Read the model definition and answer for the solid it produces. Units are mm, in the model's axes. Face numbers are marked on the shaded views. A direction names the side the tool comes from. Round coordinates to 2 decimals unless told otherwise and drop trailing zeros. Write each loop counter-clockwise with the first axis right and the second up, starting at its lowest first coordinate (ties: lowest second). Pieces come first, ordered by that corner, then holes. Notation, with made-up numbers: (22, -18) -> (51, -18) arc R26 cw to (51, -4) -> close; hole circle Ø8 at (64.5, 82). An arc over 180 degrees is marked (long way). Return JSON: item names as keys, results as strings.
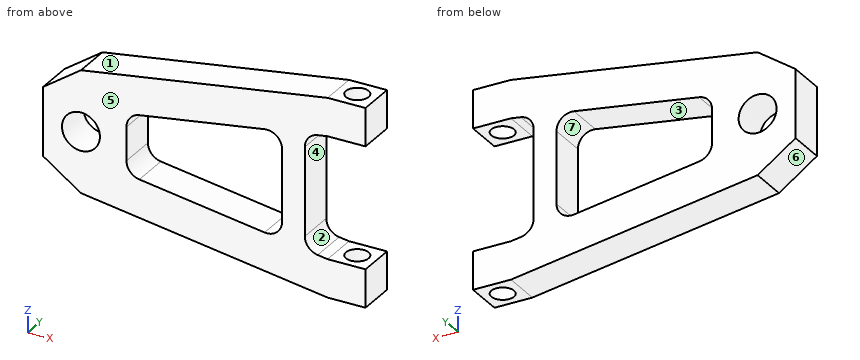
from build123d import *

# Parameters (mm, degrees)
SKETCH1_R           = 2.5
BOSS_EXTRUDE1_DEPTH = 5
SKETCH2_R           = 1.5
CUT_EXTRUDE1_DEPTH  = 46.904792778


with BuildPart() as part:
    # Sketch1 → Boss-Extrude1 (new body)
    with BuildSketch(Plane(origin=(0, 0, 0), x_dir=(1, 0, 0), z_dir=(0, 1, 0))):
        with BuildLine():
            Line((0, 8), (-5, 4.498962309))
            Line((-5, 4.498962309), (-5, -4.498962309))
            Line((-5, -4.498962309), (0, -8))
            Line((0, -8), (32.5, -13))
            Line((32.5, -13), (37.5, -13))
            Line((37.5, -13), (37.5, -8))
            Line((37.5, -8), (32.5, -8))
            Line((32.5, -8), (31.195885631, -7.79936702))
            ThreePointArc((31.195885631, -7.79936702), (29.98206905, -7.124885362), (29.5, -5.822623625))
            Line((29.5, -5.822623625), (29.5, 5.822623625))
            ThreePointArc((29.5, 5.822623625), (29.98206905, 7.124885362), (31.195885631, 7.79936702))
            Line((31.195885631, 7.79936702), (32.5, 8))
            Line((32.5, 8), (37.5, 8))
            Line((37.5, 8), (37.5, 13))
            Line((37.5, 13), (32.5, 13))
            Line((32.5, 13), (0, 8))
        make_face()
        with Locations(Location((0, 0, 0), (0, 0, 270))):
            Circle(SKETCH1_R, mode=Mode.SUBTRACT)
        with BuildLine():
            Line((6, 2.20723901), (6, -2.20723901))
            ThreePointArc((6, -2.20723901), (6.48206905, -3.509500746), (7.695885631, -4.183982405))
            Line((7.695885631, -4.183982405), (24.195885631, -6.722443943))
            ThreePointArc((24.195885631, -6.722443943), (25.802261737, -6.263631498), (26.5, -4.745700548))
            Line((26.5, -4.745700548), (26.5, 4.745700548))
            ThreePointArc((26.5, 4.745700548), (25.802261737, 6.263631498), (24.195885631, 6.722443943))
            Line((24.195885631, 6.722443943), (7.695885631, 4.183982405))
            ThreePointArc((7.695885631, 4.183982405), (6.48206905, 3.509500746), (6, 2.20723901))
        make_face(mode=Mode.SUBTRACT)
    extrude(amount=BOSS_EXTRUDE1_DEPTH)

    # Sketch2 → Cut-Extrude1 (cut, through all)
    with BuildSketch(Plane.XY.offset(13)):
        with Locations((35, 2.5)):
            Circle(SKETCH2_R)
    extrude(amount=-CUT_EXTRUDE1_DEPTH, mode=Mode.SUBTRACT)


solid = part.part
Item 1: Section A-A (y = 2.5) is taken. State how many separate pieces and enclosed holes the cut face has, then the cut area to 3 significant figures.
Worked answers:
{"separate pieces": "3", "enclosed holes": "2", "area": "478 mm2"}
Item 2: A tool of negligible diameter and unlimited length cuts with its end or side. For the marked faces 1, 2 and 3, from which of +Z, -Z, +X, -X, +Y, -Y can it reach the whole face along a straight path? Write none if from no direction.
Worked answers:
{"face 1": "+Z, -X, +Y, -Y", "face 2": "+X, +Y, -Y", "face 3": "+Y, -Y"}
Item 3: Section D-D (z = 5.25) is taken. Give the vertices of the cut face in (x, y) (3 decimals), then the cut area to 3 significant figures.
Worked answers:
{"outline": "(-3.927, 0) -> (14.625, 0) -> (14.625, 5) -> (-3.927, 5) -> close; (26.435, 0) -> (29.5, 0) -> (29.5, 5) -> (26.435, 5) -> close", "area": "108 mm2"}
Item 4: Section B-B (z = 0) is taken. Give the vertices of the cut face in (x, y), then the cut area to 3 significant figures.
Worked answers:
{"outline": "(-5, 0) -> (-2.5, 0) -> (-2.5, 5) -> (-5, 5) -> close; (2.5, 0) -> (6, 0) -> (6, 5) -> (2.5, 5) -> close; (26.5, 0) -> (29.5, 0) -> (29.5, 5) -> (26.5, 5) -> close", "area": "45.0 mm2"}
Item 5: Section C-C (x = 35) is taken. Give the vertices of the cut face in (y, z), then the cut area to 3 significant figures.
Worked answers:
{"outline": "(0, -13) -> (1, -13) -> (1, -8) -> (0, -8) -> close; (0, 8) -> (1, 8) -> (1, 13) -> (0, 13) -> close; (4, -13) -> (5, -13) -> (5, -8) -> (4, -8) -> close; (4, 8) -> (5, 8) -> (5, 13) -> (4, 13) -> close", "area": "20.0 mm2"}
Item 6: Straight lines are drawn through the part: L1, parallel to X at y = 1.1, z = 0; L2, parallel to Z at x = 33.5, y = 3.2; L3, parallel to X at y = 3.1, z = 0.5. For each, find the intervals that lie inside material, in ascending order. Write a range as [from, to].
Worked answers:
{"L1": "x = [-5, -2.5], [2.5, 6], [26.5, 29.5]", "L2": "z = [-13, -8], [8, 13]", "L3": "x = [-5, -2.45], [2.45, 6], [26.5, 29.5]"}
Item 7: Flat-ended cylindrical pins translate along their axes: pin 1 (2.5 mm diameter, centred on y = 3.5, z = 1.5, fed in from +X); pin 2 (2.5 mm diameter, centred on x = 35, y = 2.5, fed in from +Z); pin 3 (5 mm diameter, centred on x = 30.5, z = -6.5, fed in from +Y); pin 4 (1 mm diameter, centred on x = 4.5, y = 1.5, fed in from +Z). Find the tip coordinate at first contact, or state that the pin passes through.
Worked answers:
{"pin 1": "stops at x = 29.5", "pin 2": "passes through", "pin 3": "stops at y = 5", "pin 4": "stops at z = 8.77"}
Item 8: For a pull along X with two mould halves and no side action, classify the marked faces 4, 5, 6 and 7 as released by +X, released by -X, zero draft, split by the parting line, or undercut.
Worked answers:
{"face 4": "released by +X", "face 5": "zero draft", "face 6": "released by -X", "face 7": "undercut"}
